```python
from build123d import *

# Parameters (mm, degrees)
SKETCH1_W                = 83
SKETCH1_H                = 100
BOSS_EXTRUDE1_DEPTH      = 0.5
BOSS_EXTRUDE1_DEPTH_BACK = 0.5
SKETCH2_W                = 83
SKETCH2_H                = 1
BOSS_EXTRUDE2_DEPTH      = 50
BOSS_EXTRUDE2_DEPTH_BACK = 51
CUT_EXTRUDE1_REACH       = 52.5
SKETCH3_R                = 1.5


with BuildPart() as part:
    # Sketch1 → Boss-Extrude1 (new body, two sides)
    with BuildSketch(Plane(origin=(0, 0, 0), x_dir=(0, 0, -1), z_dir=(1, 0, 0))) as boss_extrude1_sk:
        Rectangle(SKETCH1_W, SKETCH1_H)
    extrude(amount=BOSS_EXTRUDE1_DEPTH)
    extrude(boss_extrude1_sk.sketch, amount=-BOSS_EXTRUDE1_DEPTH_BACK)

    # Sketch2 → Boss-Extrude2 (add, two sides)
    with BuildSketch(Plane(origin=(0.5, 0, 0), x_dir=(0, 0, -1), z_dir=(1, 0, 0))) as boss_extrude2_sk:
        Rectangle(SKETCH2_W, SKETCH2_H)
    extrude(amount=BOSS_EXTRUDE2_DEPTH)
    extrude(boss_extrude2_sk.sketch, amount=-BOSS_EXTRUDE2_DEPTH_BACK)

    # Sketch3 → Cut-Extrude1 (cut, up to next)
    with BuildSketch(Plane(origin=(0, 0.5, 0), x_dir=(1, 0, 0), z_dir=(0, 1, 0)), mode=Mode.PRIVATE) as cut_extrude1_sk1:
        with Locations((15, 31.5)):
            Circle(SKETCH3_R)
    cut_extrude1_tool1 = extrude(cut_extrude1_sk1.sketch, amount=-CUT_EXTRUDE1_REACH, mode=Mode.PRIVATE) & part.part
    add(cut_extrude1_tool1.solids().sort_by_distance((15, 0.5, -31.5))[0], mode=Mode.SUBTRACT)
    # Sketch3 → Cut-Extrude1 (cut, up to next)
    with BuildSketch(Plane(origin=(0, 0.5, 0), x_dir=(1, 0, 0), z_dir=(0, 1, 0)), mode=Mode.PRIVATE) as cut_extrude1_sk2:
        with Locations((40, 31.5)):
            Circle(SKETCH3_R)
    cut_extrude1_tool2 = extrude(cut_extrude1_sk2.sketch, amount=-CUT_EXTRUDE1_REACH, mode=Mode.PRIVATE) & part.part
    add(cut_extrude1_tool2.solids().sort_by_distance((40, 0.5, -31.5))[0], mode=Mode.SUBTRACT)
    # Sketch3 → Cut-Extrude1 (cut, up to next)
    with BuildSketch(Plane(origin=(0, 0.5, 0), x_dir=(1, 0, 0), z_dir=(0, 1, 0)), mode=Mode.PRIVATE) as cut_extrude1_sk3:
        with Locations((-40, 31.5)):
            Circle(SKETCH3_R)
    cut_extrude1_tool3 = extrude(cut_extrude1_sk3.sketch, amount=-CUT_EXTRUDE1_REACH, mode=Mode.PRIVATE) & part.part
    add(cut_extrude1_tool3.solids().sort_by_distance((-40, 0.5, -31.5))[0], mode=Mode.SUBTRACT)
    # Sketch3 → Cut-Extrude1 (cut, up to next)
    with BuildSketch(Plane(origin=(0, 0.5, 0), x_dir=(1, 0, 0), z_dir=(0, 1, 0)), mode=Mode.PRIVATE) as cut_extrude1_sk4:
        with Locations((-15, 31.5)):
            Circle(SKETCH3_R)
    cut_extrude1_tool4 = extrude(cut_extrude1_sk4.sketch, amount=-CUT_EXTRUDE1_REACH, mode=Mode.PRIVATE) & part.part
    add(cut_extrude1_tool4.solids().sort_by_distance((-15, 0.5, -31.5))[0], mode=Mode.SUBTRACT)


solid = part.part
```
Geometry check sheet. Reference: the model listing, model coordinates, mm. A direction names the side the tool comes from. Coordinates: 2 decimals unless noted, no trailing zeros. Order: outer loops, then holes, each group sorted by start corner. A loop starts at its lowest first (then second) coordinate and runs counter-clockwise, first axis right, second up.
Item 1: Section check C-C (z = -3). Enter the section's corners in (x, y).
Item 2: Section check A-A (x = 40). Enter the section's corners in (y, z), plus the area to 3 significant figures.
Item 3: Depth check by flat-ended pin: pin 1 (8 mm diameter, centred on x = -17, z = 21.5, fed in from -Y); pin 2 (15 mm diameter, centred on x = 17, z = -17, fed in from +Y); pin 3 (25 mm diameter, centred on y = -24.5, z = 19, fed in from -X). Enter the tip coordinate at first touch or a pass-through.
Item 4: Mould release check, pull along Z, two halves, no side actions. Record for faces 1 (the flat face through (0, 0, -41.5)), 2 (the flat face through (0, 0, 41.5)), 3 (the flat face through (0.5, -25, 1)), 4 (the cylindrical face through (-16.5, 0.01, -31.57)): released by +Z, released by -Z, zero draft, split by the parting line, or undercut.
Item 5: Section check B-B (z = -31.5). Enter the section's corners in (x, y), plus the area to 3 significant figures.
Item 6: Scan lines: line 1 along X through (y, z) = (0, -31.5); line 2 along Z through (x, y) = (40, 0.1); line 3 along X through (y, z) = (0, -31). Record each from-to range of solid material in increasing order.
Item 7: Section check D-D (y = -12). Enter the section's corners in (x, z), plus the area to 3 significant figures.
Item 8: Tool access check on faces 5 (the flat face through (-0.5, 26, 1)), 6 (the flat face through (25, 0.5, 1)), 7 (the flat face through (-25, -0.5, 1)). Record the directions out of +Z, -Z, +X, -X, +Y, -Y that give a thin tool (end or side, any length) a straight path to the whole face; none if there is none.
Check sheet entries:
1. outline: (-50.5, -0.5) - (-0.5, -0.5) - (-0.5, -50) - (0.5, -50) - (0.5, -0.5) - (50.5, -0.5) - (50.5, 0.5) - (0.5, 0.5) - (0.5, 50) - (-0.5, 50) - (-0.5, 0.5) - (-50.5, 0.5) - close
2. outline: (-0.5, -41.5) - (0.5, -41.5) - (0.5, -33) - (-0.5, -33) - close; (-0.5, -30) - (0.5, -30) - (0.5, 41.5) - (-0.5, 41.5) - close
2. area: 80.0 mm2
3. pin 1: stops at y = -0.5
3. pin 2: stops at y = 0.5
3. pin 3: stops at x = -0.5
4. face 1: released by -Z
4. face 2: released by +Z
4. face 3: zero draft
4. face 4: undercut
5. outline: (-50.5, -0.5) - (-41.5, -0.5) - (-41.5, 0.5) - (-50.5, 0.5) - close; (-38.5, -0.5) - (-16.5, -0.5) - (-16.5, 0.5) - (-38.5, 0.5) - close; (-13.5, -0.5) - (-0.5, -0.5) - (-0.5, -50) - (0.5, -50) - (0.5, -0.5) - (13.5, -0.5) - (13.5, 0.5) - (0.5, 0.5) - (0.5, 50) - (-0.5, 50) - (-0.5, 0.5) - (-13.5, 0.5) - close; (16.5, -0.5) - (38.5, -0.5) - (38.5, 0.5) - (16.5, 0.5) - close; (41.5, -0.5) - (50.5, -0.5) - (50.5, 0.5) - (41.5, 0.5) - close
5. area: 188 mm2
6. line 1: x = -50.5 to -41.5, -38.5 to -16.5, -13.5 to 13.5, 16.5 to 38.5, 41.5 to 50.5
6. line 2: z = -41.5 to -33, -30 to 41.5
6. line 3: x = -50.5 to -41.41, -38.59 to -16.41, -13.59 to 13.59, 16.41 to 38.59, 41.41 to 50.5
7. outline: (-0.5, -41.5) - (0.5, -41.5) - (0.5, 41.5) - (-0.5, 41.5) - close
7. area: 83.0 mm2
8. face 5: +Z, -Z, -X, +Y
8. face 6: +Z, -Z, +X, +Y
8. face 7: +Z, -Z, -X, -Y
